Geometry: final body of the model. Coordinates: model frame, mm. Round coordinates to 2 decimals unless told otherwise and drop trailing zeros. Loops run counter-clockwise (first coordinate to the right, second up) from the corner with the lowest first, then second, coordinate; pieces in that order, holes last. Notation, with made-up numbers: (61.5, 61) - (106.5, 61) arc R11 cw to (106.5, 68) - close; hole circle Ø7 at (-34.5, 60). An arc over 180 degrees is marked (long way). Use CSV: the item, a comma, the result in double quotes.
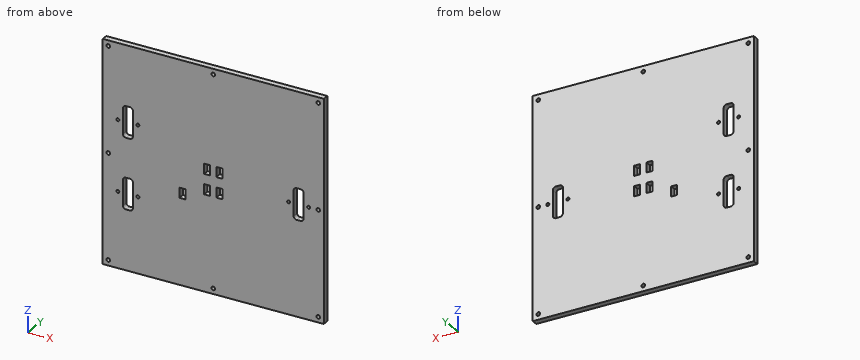
from build123d import *

# Parameters (mm, degrees)
SKETCH1_W                  = 220
SKETCH1_H                  = 220
BOSS_EXTRUDE1_DEPTH        = 6
SKETCH2_R                  = 1.5
SKETCH2_W                  = 10
SKETCH2_H                  = 31
CUT_EXTRUDE1_DEPTH         = 7
FILLET1_R                  = 3
SKETCH5_R                  = 1.5
SKETCH5_W                  = 10
SKETCH5_H                  = 31
CUT_EXTRUDE3_DEPTH         = 7
FILLET2_R                  = 3
SKETCH7_R                  = 1.5
SKETCH7_W                  = 10
SKETCH7_H                  = 31
CUT_EXTRUDE4_DEPTH         = 7
FILLET3_R                  = 3
F_3_6_3_6_DIAMETER_HOLE1_D = 3.6
SKETCH6_W                  = 10
SKETCH6_H                  = 6
CUT_EXTRUDE12_DEPTH        = 4
SKETCH61_W                 = 10
SKETCH61_H                 = 6
CUT_EXTRUDE13_DEPTH        = 4
SKETCH65_W                 = 10
SKETCH65_H                 = 6
CUT_EXTRUDE16_DEPTH        = 4
CUT_EXTRUDE16_DEPTH_BACK   = 4


with BuildPart() as part:
    # Sketch1 → Boss-Extrude1 (new body)
    with BuildSketch(Plane(origin=(0, 0, 0), x_dir=(1, 0, 0), z_dir=(0, 1, 0))):
        Rectangle(SKETCH1_W, SKETCH1_H)
    extrude(amount=BOSS_EXTRUDE1_DEPTH)

    # Sketch2 → Cut-Extrude1 (cut, through all)
    with BuildSketch(Plane(origin=(0, 6, 0), x_dir=(1, 0, 0), z_dir=(0, 1, 0))):
        with Locations((-95, 35)):
            Circle(SKETCH2_R)
        with Locations((-75, 35)):
            Circle(SKETCH2_R)
        with Locations((-85, 35)):
            Rectangle(SKETCH2_W, SKETCH2_H)
    extrude(amount=-CUT_EXTRUDE1_DEPTH, mode=Mode.SUBTRACT)

    # Fillet1
    fillet1_edges = [part.edges().sort_by_distance(p)[0] for p in [
        (-80, 3, -50.5),
        (-80, 3, -19.5),
        (-90, 3, -19.5),
        (-90, 3, -50.5),
    ]]
    fillet(fillet1_edges, radius=FILLET1_R)

    # Sketch5 → Cut-Extrude3 (cut, through all)
    with BuildSketch(Plane(origin=(45.510619452, 6, 46.414764374), x_dir=(1, 0, 0), z_dir=(0, 1, 0))):
        with Locations((-140.510619452, 11.414764374)):
            Circle(SKETCH5_R)
        with Locations((-120.510619452, 11.414764374)):
            Circle(SKETCH5_R)
        with Locations((-130.510619452, 11.414764374)):
            Rectangle(SKETCH5_W, SKETCH5_H)
    extrude(amount=-CUT_EXTRUDE3_DEPTH, mode=Mode.SUBTRACT)

    # Fillet2
    fillet2_edges = [part.edges().sort_by_distance(p)[0] for p in [
        (-80, 3, 19.5),
        (-80, 3, 50.5),
        (-90, 3, 50.5),
        (-90, 3, 19.5),
    ]]
    fillet(fillet2_edges, radius=FILLET2_R)

    # Sketch7 → Cut-Extrude4 (cut, through all)
    with BuildSketch(Plane(origin=(105.138163787, 6, 83.209962186), x_dir=(1, 0, 0), z_dir=(0, 1, 0))):
        with Locations((-30.138163787, 83.209962186)):
            Circle(SKETCH7_R)
        with Locations((-10.138163787, 83.209962186)):
            Circle(SKETCH7_R)
        with Locations((-20.138163787, 83.209962186)):
            Rectangle(SKETCH7_W, SKETCH7_H)
    extrude(amount=-CUT_EXTRUDE4_DEPTH, mode=Mode.SUBTRACT)

    # Fillet3
    fillet3_edges = [part.edges().sort_by_distance(p)[0] for p in [
        (90, 3, -15.5),
        (90, 3, 15.5),
        (80, 3, 15.5),
        (80, 3, -15.5),
    ]]
    fillet(fillet3_edges, radius=FILLET3_R)

    # Ø3.6 (3.6) Diameter Hole1 (through all)
    with Locations(Plane(origin=(0, 6, 0), x_dir=(1, 0, 0), z_dir=(0, 1, 0))):
        with Locations((-104.5, -104.5), (0, -104.5), (104.5, -104.5), (104.5, 0), (104.5, 104.5), (0, 104.5), (-104.5, 104.5), (-104.5, 0)):
            Hole(F_3_6_3_6_DIAMETER_HOLE1_D / 2)

    # Sketch6 → Cut-Extrude12 (cut, symmetric)
    with BuildSketch(Plane(origin=(-38, 3, -10.767778608), x_dir=(0, 0, 1), z_dir=(0, -1, 0))):
        with Locations((0.767778608, -44)):
            Rectangle(SKETCH6_W, SKETCH6_H)
    cut_extrude12 = extrude(amount=CUT_EXTRUDE12_DEPTH, both=True, mode=Mode.SUBTRACT)

    # Sketch61 → Cut-Extrude13 (cut, symmetric)
    with BuildSketch(Plane(origin=(-38, 3, 9.232221392), x_dir=(0, 0, 1), z_dir=(0, -1, 0))):
        with Locations((0.767778608, -44)):
            Rectangle(SKETCH61_W, SKETCH61_H)
    cut_extrude13 = extrude(amount=CUT_EXTRUDE13_DEPTH, both=True, mode=Mode.SUBTRACT)

    # Mirror1: Cut-Extrude12, Cut-Extrude13 across plane
    add(cut_extrude12.mirror(Plane(origin=(0, 0, 0), x_dir=(0, 0, 1), z_dir=(1, 0, 0))), mode=Mode.SUBTRACT)
    add(cut_extrude13.mirror(Plane(origin=(0, 0, 0), x_dir=(0, 0, 1), z_dir=(1, 0, 0))), mode=Mode.SUBTRACT)

    # Sketch65 → Cut-Extrude16 (cut, two sides)
    with BuildSketch(Plane(origin=(-74.75, 3, -20.767778608), x_dir=(0, 0, 1), z_dir=(0, -1, 0))) as cut_extrude16_sk:
        with Locations((0.767778608, -44)):
            Rectangle(SKETCH65_W, SKETCH65_H)
    extrude(amount=CUT_EXTRUDE16_DEPTH, mode=Mode.SUBTRACT)
    extrude(cut_extrude16_sk.sketch, amount=-CUT_EXTRUDE16_DEPTH_BACK, mode=Mode.SUBTRACT)


solid = part.part
Item 1: Section B-B on y = 2.75. Give the number of separate pieces and of enclosed holes in the cut face, plus the area to 3 significant figures.
Final values:
separate pieces,"1"
enclosed holes,"22"
area,"47,100 mm²"
Item 2: Material intervals for line 1 (Z direction, x = 104.5, y = 2.2); line 2 (Z direction, x = -95, y = 1.6), sorted ascending.
Final values:
line 1,"z = -110 to -106.3, -102.7 to -1.8, 1.8 to 102.7, 106.3 to 110"
line 2,"z = -110 to -36.5, -33.5 to 33.5, 36.5 to 110"
Item 3: Section A-A on z = 44. Return the cut outline in (x, y), plus the area to 3 significant figures.
Final values:
outline,"(-110, 0) - (-90, 0) - (-90, 6) - (-110, 6) - close; (-80, 0) - (110, 0) - (110, 6) - (-80, 6) - close"
area,"1,260 mm²"
Item 4: Pin query (flat end, axial travel): P1, Ø1.8, axis at x = -75, z = 35, coming from the -Y side. Return the tip coordinate at first contact, or that it passes through.
Final values:
P1,"passes through"
